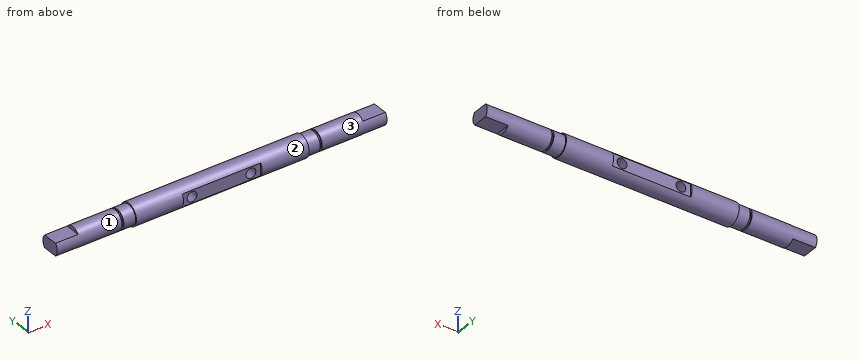
```python
from build123d import *

# Parameters (mm, degrees)
CORTAR_EXTRUIR1_START      = -23
CORTAR_EXTRUIR1_DEPTH      = 23
CORTAR_EXTRUIR2_DEPTH      = 238.026751177
CORTAR_EXTRUIR2_DEPTH_BACK = 238.026751177
CROQUIS3_W                 = 80
CROQUIS3_H                 = 4
CROQUIS4_R                 = 5
CORTAR_EXTRUIR3_DEPTH      = 238.628373184


with BuildPart() as part:
    # Croquis1 → Revolución1 (revolve)
    with BuildSketch(Plane.XY, mode=Mode.PRIVATE) as revoluci_n1_sk:
        Polygon((-19.494808808, 11.1125), (68.505191192, 11.1125), (68.505191192, 0), (-99.494808808, 0), (-99.494808808, 10), (-33.494808808, 10), (-33.494808808, 8.5), (-31.494808808, 8.5), (-31.494808808, 10), (-19.494808808, 10), align=None)
    revoluci_n1 = revolve(revoluci_n1_sk.sketch.rotate(Axis((70.414965315, 0, 0), (-1, 0, 0)), 90), axis=Axis((70.414965315, 0, 0), (-1, 0, 0)))

    # Croquis2 → Cortar-Extruir1 (cut)
    with BuildSketch(Plane.ZY.offset(99.494808808).offset(CORTAR_EXTRUIR1_START)):
        with BuildLine():
            Line((-6.278365003, -7.783452504), (-6.278365003, 7.783452504))
            ThreePointArc((-6.278365003, 7.783452504), (-10, 0), (-6.278365003, -7.783452504))
        make_face()
        with BuildLine():
            Line((6.278365003, -7.783452504), (6.278365003, 7.783452504))
            ThreePointArc((6.278365003, 7.783452504), (10, 0), (6.278365003, -7.783452504))
        make_face()
    cortar_extruir1 = extrude(amount=CORTAR_EXTRUIR1_DEPTH, mode=Mode.SUBTRACT)

    # Simetría2: Revolución1, Cortar-Extruir1 across plane
    add(revoluci_n1.mirror(Plane(origin=(68.505191192, 11.1125, 0), x_dir=(0, 0, 1), z_dir=(1, 0, 0))))
    add(cortar_extruir1.mirror(Plane(origin=(68.505191192, 11.1125, 0), x_dir=(0, 0, 1), z_dir=(1, 0, 0))), mode=Mode.SUBTRACT)

    # Croquis3 → Cortar-Extruir2 (cut, two sides: drawn at the far end of the back side and taken through both)
    with BuildSketch(Plane.XY.offset(-CORTAR_EXTRUIR2_DEPTH_BACK)):
        with Locations((68.505191192, 11.1125)):
            Rectangle(CROQUIS3_W, CROQUIS3_H)
        with Locations((68.505191192, -11.1125)):
            Rectangle(CROQUIS3_W, CROQUIS3_H)
    extrude(amount=CORTAR_EXTRUIR2_DEPTH + CORTAR_EXTRUIR2_DEPTH_BACK, mode=Mode.SUBTRACT)

    # Croquis4 → Cortar-Extruir3 (cut, through all)
    with BuildSketch(Plane(origin=(0, 9.1125, 0), x_dir=(1, 0, 0), z_dir=(0, 1, 0))):
        with Locations(Location((38.505191192, 0, 0), (0, 0, 270))):
            Circle(CROQUIS4_R)
        with Locations(Location((98.505191192, 0, 0), (0, 0, 270))):
            Circle(CROQUIS4_R)
    extrude(amount=-CORTAR_EXTRUIR3_DEPTH, mode=Mode.SUBTRACT)


solid = part.part
```
Input: part model. Units: mm. Frame: model coordinates. Face numbers are marked on the shaded views. A direction names the side the tool comes from. Give positions to 0.01 mm unless a question says otherwise; leave off trailing zeros. Loops run counter-clockwise (first coordinate to the right, second up) from the corner with the lowest first, then second, coordinate; pieces in that order, holes last. Notation, with made-up numbers: (6.5, 74.25) -> (14.5, 74.25) arc R31 cw to (14.5, 109.25) -> close; hole circle Ø4 at (69.25, 51.5). An arc over 180 degrees is marked (long way). Use a Markdown table: item, result.
Q1. First-contact query: P1, Ø8, axis at x = -32, z = -5.5, coming from the +Y side; P2, Ø2, axis at x = 64, y = -7.5, coming from the -Z side; P3, Ø5, axis at x = 164.5, y = 3, coming from the +Z side. Flat tips, straight axial feed; report the tip coordinate or a pass-through.
Entries:
| item | result |
|---|---|
| P1 | stops at y = 9.88 |
| P2 | stops at z = -9.01 |
| P3 | stops at z = 9.99 |
Q2. Access query for the marked faces 1, 2 and 3. Directions: +Z, -Z, +X, -X, +Y, -Y. A direction counts if a zero-diameter tool reaches every point of the face in a straight line with its end or side. Return the directions, or none.
Entries:
| item | result |
|---|---|
| face 1 | -X |
| face 2 | +X, -X |
| face 3 | +X |
Q3. Ray query, probe 1 along X at (y, z) = (-4.5, 0); probe 2 along X at (y, z) = (0.5, -0.75); probe 3 along Z at (x, y) = (-41, 6.25). Return the intervals inside material, ascending. Write a range as from..to.
Entries:
| item | result |
|---|---|
| probe 1 | x = -99.49..33.51, 43.51..93.51, 103.51..236.51 |
| probe 2 | x = -99.49..33.56, 43.45..93.56, 103.45..236.51 |
| probe 3 | z = -7.81..7.81 |
Q4. Section query A-A, the plane z = 0. State how many separate pieces and enclosed holes the cut face has, plus the area to 3 significant figures.
Entries:
| item | result |
|---|---|
| separate pieces | 3 |
| enclosed holes | 0 |
| area | 6,420 mm² |
Q5. Section query B-B, the plane x = -47.5. Return the cut outline in (y, z), plus the area to 3 significant figures.
Entries:
| item | result |
|---|---|
| outline | circle Ø20 at (0, 0) |
| area | 314 mm² |
